from build123d import *

# Parameters (mm, degrees)
SKETCH1_W                 = 60
SKETCH1_H                 = 80
BOSS_EXTRUDE1_DEPTH       = 4
SKETCH2_W                 = 60
SKETCH2_H                 = 10
BOSS_EXTRUDE2_DEPTH       = 6
F_8_0MM_DOWEL_HOLE1_D     = 8
F_8_0MM_DOWEL_HOLE1_DEPTH = 6
CUT_EXTRUDE1_DEPTH        = 101.498756211


with BuildPart() as part:
    # Sketch1 → Boss-Extrude1 (new body)
    with BuildSketch(Plane(origin=(0, 0, 0), x_dir=(1, 0, 0), z_dir=(0, 1, 0))):
        with Locations((30, 40)):
            Rectangle(SKETCH1_W, SKETCH1_H)
    extrude(amount=BOSS_EXTRUDE1_DEPTH)

    # Sketch2 → Boss-Extrude2 (add)
    with BuildSketch(Plane.XY):
        with Locations((30, 5)):
            Rectangle(SKETCH2_W, SKETCH2_H)
    extrude(amount=-BOSS_EXTRUDE2_DEPTH)

    # Ø8.0mm Dowel Hole1
    with Locations(Plane(origin=(0, 4, 0), x_dir=(1, 0, 0), z_dir=(0, 1, 0))):
        with Locations((30, 70)):
            Hole(F_8_0MM_DOWEL_HOLE1_D / 2, depth=F_8_0MM_DOWEL_HOLE1_DEPTH)

    # Sketch6 → Cut-Extrude1 (cut, through all)
    with BuildSketch(Plane.XZ):
        with BuildLine():
            Line((25.84299387, -39.154412182), (41.293514764, -34.997321359))
            ThreePointArc((41.293514764, -34.997321359), (43.744466229, -36.409000118), (42.33278747, -38.859951582))
            Line((42.33278747, -38.859951582), (26.882266576, -43.017042406))
            ThreePointArc((26.882266576, -43.017042406), (24.431315112, -41.605363647), (25.84299387, -39.154412182))
        make_face()
    extrude(amount=-CUT_EXTRUDE1_DEPTH, mode=Mode.SUBTRACT)


solid = part.part
The model under review builds one solid part; all positions refer to its coordinate system, in mm. A direction names the side the tool comes from. Give positions to 0.01 mm unless a question says otherwise; leave off trailing zeros. Loops run counter-clockwise (first coordinate to the right, second up) from the corner with the lowest first, then second, coordinate; pieces in that order, holes last. Notation, with made-up numbers: (87, 34.25) -> (145, 34.25) arc R29 ccw to (145, 73.25) -> close; hole circle Ø4 at (-34, -2.5). An arc over 180 degrees is marked (long way). Answer as a JSON object with one key per item and string values. Group by question number.
Q1. Take a section at B-B (z = -70). Write out the cut boundary in (x, y), plus the area to 3 significant figures.
Q2. Take a section at A-A (y = 2.5). Write out the cut boundary in (x, z), plus the area to 3 significant figures.
Q3. Take a section at C-C (x = 30). Write out the cut boundary in (y, z).
Q4. Wall thickness on line 1 along Z through (x, y) = (30, 2.8); line 2 along Z through (x, y) = (33, 0.75); line 3 along X through (y, z) = (2.25, -70): over which ranges is each line inside the solid? List them lowest first.
Q5. Draft analysis for pull direction X (two halves, no side actions). For faces 4 (the cylindrical face through (43.733, 1.972, -36.367)), 5 (the flat face through (23, 0, -41)), 6 (the flat face through (60, 3, -39)), state which applies: pulls with the +X half, pulls with the -X half, needs draft (parallel to the pull), parting line crosses it, or undercut.
Q6. Tool access review of faces 1 (the flat face through (30, 7, -6)), 2 (the flat face through (34.72, 1.97, -40.91)), 3 (the flat face through (30, 5, 0)): name each direction out of +Z, -Z, +X, -X, +Y, -Y from which nothing blocks a thin tool from reaching the whole face with its end or side.
Q7. Take a section at D-D (x = 56). Write out the cut boundary in (y, z).
Q8. Insertion check: pin 1 (5 mm diameter, centred on x = 25, y = 8, fed in from -Z). The pin has a flat end and moves straight along its axis. Give the tip position at first contact, or say it passes through.
Answer below:
{
 "1": {"outline": "(0, 0) -> (26, 0) -> (26, 4) -> (0, 4) -> close; (34, 0) -> (60, 0) -> (60, 4) -> (34, 4) -> close", "area": "208 mm2"},
 "2": {"outline": "(0, -80) -> (60, -80) -> (60, 0) -> (0, 0) -> close; hole (25.84, -39.15) arc R2 ccw to (26.88, -43.02) -> (42.33, -38.86) arc R2 ccw to (41.29, -35) -> close; hole circle Ø8 at (30, -70)", "area": "4,670 mm2"},
 "3": {"outline": "(0, -80) -> (4, -80) -> (4, -74) -> (0, -74) -> close; (0, -66) -> (4, -66) -> (4, -42.18) -> (0, -42.18) -> close; (0, -38.04) -> (4, -38.04) -> (4, -6) -> (10, -6) -> (10, 0) -> (0, 0) -> close"},
 "4": {"line 1": "z = -80 to -74, -66 to -42.18, -38.04 to 0", "line 2": "z = -80 to -72.65, -67.35 to -41.37, -37.23 to 0", "line 3": "x = 0 to 26, 34 to 60"},
 "5": {"face 4": "undercut", "face 5": "needs draft", "face 6": "pulls with the +X half"},
 "6": {"face 1": "-Z, +X, -X, +Y", "face 2": "+Y, -Y", "face 3": "+Z, +X, -X, +Y, -Y"},
 "7": {"outline": "(0, -80) -> (4, -80) -> (4, -6) -> (10, -6) -> (10, 0) -> (0, 0) -> close"},
 "8": {"pin 1": "stops at z = -6"}
}
